Build history of the part. All positions in model axes, mm. Face numbers are marked on the shaded views. A direction names the side the tool comes from. Round coordinates to 2 decimals unless told otherwise and drop trailing zeros. Write each loop counter-clockwise with the first axis right and the second up, starting at its lowest first coordinate (ties: lowest second). Pieces come first, ordered by that corner, then holes.
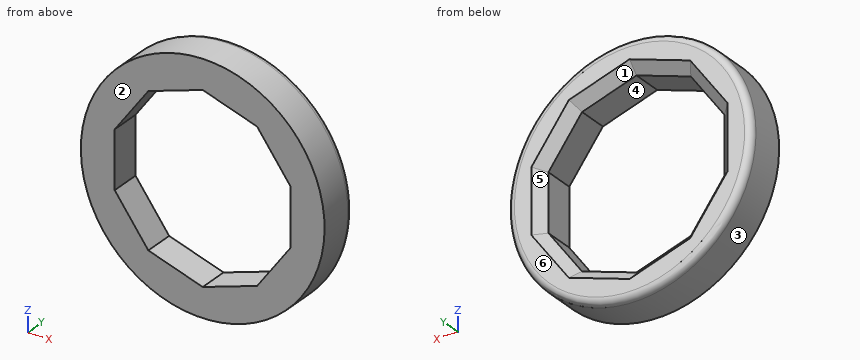
from build123d import *

# Parameters (mm, degrees)
SKETCH1_R           = 36
BOSS_EXTRUDE1_DEPTH = 12
FILLET1_R           = 2
CHAMFER1_SIZE       = 3


with BuildPart() as part:
    # Sketch1 → Boss-Extrude1 (new body)
    with BuildSketch(Plane(origin=(0, 0, 0), x_dir=(1, 0, 0), z_dir=(0, 1, 0))):
        with Locations(Location((0, 0, 0), (0, 0, 270))):
            Circle(SKETCH1_R)
        Polygon((16.068883707, 22.116921017), (0, 27.33801783), (-16.068883707, 22.116921017), (-26, 8.447912102), (-26, -8.447912102), (-16.068883707, -22.116921017), (0, -27.33801783), (16.068883707, -22.116921017), (26, -8.447912102), (26, 8.447912102), align=None, mode=Mode.SUBTRACT)
    extrude(amount=BOSS_EXTRUDE1_DEPTH)

    # Fillet1
    fillet1_edges = [part.edges().sort_by_distance(p)[0] for p in [
        (0, 12, -36),
    ]]
    fillet(fillet1_edges, radius=FILLET1_R)

    # Chamfer1
    chamfer1_edges = [part.edges().sort_by_distance(p)[0] for p in [
        (21.034441854, 12, -15.28241656),
        (8.034441854, 12, -24.727469424),
        (-8.034441854, 12, -24.727469424),
        (-21.034441854, 12, -15.28241656),
        (-26, 12, 0),
        (-21.034441854, 12, 15.28241656),
        (-8.034441854, 12, 24.727469424),
        (8.034441854, 12, 24.727469424),
        (21.034441854, 12, 15.28241656),
        (26, 12, 0),
    ]]
    chamfer(chamfer1_edges, length=CHAMFER1_SIZE)


solid = part.part
1) Slice it at A-A (z = 0). Write the cut outline in (x, y), plus the area to 3 significant figures.
Results:
outline: (-36, 0) - (-26, 0) - (-26, 9) - (-29, 12) - (-34, 12) arc R2 ccw to (-36, 10) - close; (26, 0) - (36, 0) - (36, 10) arc R2 ccw to (34, 12) - (29, 12) - (26, 9) - close
area: 229 mm2
2) Mould opens along X. For the marked faces 1, 2 and 3 say: released by +X, released by -X, zero draft, split by the parting line, or undercut.
Results:
face 1: undercut
face 2: zero draft
face 3: split by the parting line
3) Pin check, flat tips, straight feed: pin 1 Ø2.5 at (y, z) = (4, -1) entering from +X; pin 2 Ø5 at (x, y) = (-13.5, 3) entering from -Z; pin 3 Ø2 at (y, z) = (10, 20.5) entering from +X; pin 4 Ø6 at (x, y) = (2, 10.5) entering from -Z. Stop position of each tip, or through.
Results:
pin 1: stops at x = 36
pin 2: stops at z = -34.28
pin 3: stops at x = 30.26
pin 4: stops at z = -36
4) Which spindle directions (+Z, -Z, +X, -X, +Y, -Y) get a long thin tool onto all of the face, cutting with end or side? Do the marked faces 4, 5 and 6. Say none if no direction does.
Results:
face 4: +Y, -Y
face 5: +Y
face 6: +Z, -Z, +X, -X, +Y
5) Wall check: L1, parallel to X at y = 6.25, z = 0.5; L2, parallel to X at y = 11, z = -8.5; L3, parallel to Z at x = -21.5, y = 8.5. Give the ranges that are in metal, low to high.
Results:
L1: x = -36 to -26, 26 to 36
L2: x = -34.71 to -28, 28 to 34.71
L3: z = -28.87 to -14.64, 14.64 to 28.87
